Could you check a few things on this model? Use its own coordinates, in mm. Face numbers are marked on the shaded views. Round coordinates to 2 decimals unless told otherwise and drop trailing zeros. Put each result on its own line as item: value.
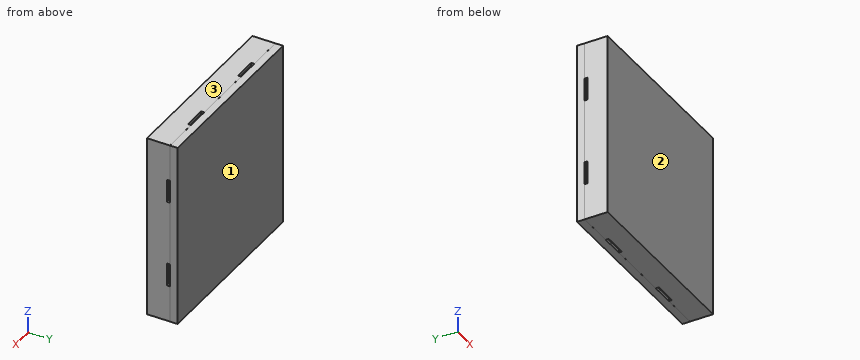
from build123d import *

# Parameters (mm, degrees)
SKETCH_1_W          = 600
SKETCH_1_H          = 600
EXTRUDE_1_DEPTH     = 200
CUT_EXTRUDE_1_DEPTH = 20
CUT_EXTRUDE_2_DEPTH = 20


with BuildPart() as part:
    # 草图1 → 凸台-拉伸1 (new body)
    with BuildSketch(Plane(origin=(0, 0, 0), x_dir=(1, 0, 0), z_dir=(0, 1, 0))):
        with Locations((-300, -300)):
            Rectangle(SKETCH_1_W, SKETCH_1_H)
    extrude(amount=EXTRUDE_1_DEPTH)

    # 草图2 → 切除-拉伸1 (cut)
    with BuildSketch(Plane.ZY.offset(600)):
        Polygon((600, 150.2), (0, 150.2), (0, 150), (210, 150), (210, 130), (360, 130), (360, 150), (600, 150), align=None)
    extrude(amount=-CUT_EXTRUDE_1_DEPTH, mode=Mode.SUBTRACT)

    # 草图3 → 切除-拉伸2 (cut)
    with BuildSketch(Plane.XY.offset(600)):
        Polygon((-580, 150.2), (-580, 150), (-360, 150), (-360, 130), (-210, 130), (-210, 150), (0, 150), (0, 150.2), align=None)
    extrude(amount=-CUT_EXTRUDE_2_DEPTH, mode=Mode.SUBTRACT)

    # 镜向1: part across plane


with BuildPart() as part_1:
    add(part.part)
    add(part.part.mirror(Plane(origin=(0, 200, 0), x_dir=(1, 0, 0), z_dir=(0, 0, 1))))

    # 镜向2: part across plane


with BuildPart() as part_2:
    add(part_1.part)
    add(part_1.part.mirror(Plane(origin=(0, 200, 0), x_dir=(0, 0, 1), z_dir=(-1, 0, 0))))


solid = part_2.part
(1) Please list where this line runs through material, in increasing order: probe 1 along X at (y, z) = (134.5, 314.5). Write a range as from..to.
Values found:
probe 1: x = -580..580
(2) If we mould it in two halves opening along Y, with no side actions, what happens to the marked faces 1, 2 and 3? For each: pulls with the +Y half, pulls with the -Y half, needs draft (parallel to the pull), parting line crosses it, or undercut.
Values found:
face 1: pulls with the +Y half
face 2: pulls with the -Y half
face 3: needs draft
(3) I'm going to push a flat-ended pin straight in: pin 1 (3 mm diameter, centred on x = -315, y = 134.5, fed in from -Z). Where does the tip first touch, or does it pass through?
Values found:
pin 1: stops at z = -580
